Check sheet for the modelled part. Datum: model origin and axes. Units: mm. A direction names the side the tool comes from. Give positions to 0.01 mm unless a question says otherwise; leave off trailing zeros. Order: outer loops, then holes, each group sorted by start corner. A loop starts at its lowest first (then second) coordinate and runs counter-clockwise, first axis right, second up. Notation, with made-up numbers: (61, -35) - (76, -35) arc R10 ccw to (76, -26) - close; hole circle Ø4 at (28.5, 10.25). An arc over 180 degrees is marked (long way). Answer in a Markdown table with one row per item.
from build123d import *

# Parameters (mm, degrees)
SKETCH014_R     = 50
SKETCH014_R_2   = 31
SKETCH014_R_3   = 1.7
PAD014_DEPTH    = 8
SKETCH015_R     = 32.6
POCKET_DEPTH    = 7
SKETCH016_R     = 2.5
POCKET001_DEPTH = 7
SKETCH017_R     = 3
POCKET002_DEPTH = 4


with BuildPart() as part:
    # Sketch014 → Pad014 (new body)
    with BuildSketch(Plane.YZ):
        Circle(SKETCH014_R)
        Circle(SKETCH014_R_2, mode=Mode.SUBTRACT)
        with Locations((46, 0)):
            Circle(SKETCH014_R_3, mode=Mode.SUBTRACT)
        with Locations((-46, 0)):
            Circle(SKETCH014_R_3, mode=Mode.SUBTRACT)
        with Locations((0, -46)):
            Circle(SKETCH014_R_3, mode=Mode.SUBTRACT)
        with Locations((0, 46)):
            Circle(SKETCH014_R_3, mode=Mode.SUBTRACT)
        with Locations((-39.837169, 23)):
            Circle(SKETCH014_R_3, mode=Mode.SUBTRACT)
        with Locations((-23, 39.837169)):
            Circle(SKETCH014_R_3, mode=Mode.SUBTRACT)
        with Locations((39.837169, 23)):
            Circle(SKETCH014_R_3, mode=Mode.SUBTRACT)
        with Locations((39.837169, -23)):
            Circle(SKETCH014_R_3, mode=Mode.SUBTRACT)
        with Locations((23, -39.837169)):
            Circle(SKETCH014_R_3, mode=Mode.SUBTRACT)
        with Locations((23, 39.837169)):
            Circle(SKETCH014_R_3, mode=Mode.SUBTRACT)
        with Locations((-23, -39.837169)):
            Circle(SKETCH014_R_3, mode=Mode.SUBTRACT)
        with Locations((-39.837169, -23)):
            Circle(SKETCH014_R_3, mode=Mode.SUBTRACT)
    extrude(amount=PAD014_DEPTH)

    # Sketch015 (on DatumPlane) → Pocket (cut)
    with BuildSketch(Plane(origin=(0, 0, 0), x_dir=(0, 1, 0), z_dir=(-1, 0, 0))):
        Circle(SKETCH015_R)
    extrude(amount=-POCKET_DEPTH, mode=Mode.SUBTRACT)

    # Sketch016 (on DatumPlane) → Pocket001 (cut)
    with BuildSketch(Plane(origin=(0, 0, 0), x_dir=(0, 1, 0), z_dir=(-1, 0, 0))):
        with Locations((0, 35)):
            Circle(SKETCH016_R)
        with Locations((-35, 0)):
            Circle(SKETCH016_R)
        with Locations((0, -35)):
            Circle(SKETCH016_R)
        with Locations((35, 0)):
            Circle(SKETCH016_R)
        with Locations((24.748737, -24.748737)):
            Circle(SKETCH016_R)
        with Locations((-24.748737, -24.748737)):
            Circle(SKETCH016_R)
        with Locations((-24.748737, 24.748737)):
            Circle(SKETCH016_R)
        with Locations((24.748737, 24.748737)):
            Circle(SKETCH016_R)
    extrude(amount=-POCKET001_DEPTH, mode=Mode.SUBTRACT)

    # Sketch017 (on DatumPlane) → Pocket002 (cut)
    with BuildSketch(Plane.YZ.offset(8)):
        with Locations((-46, 0)):
            Circle(SKETCH017_R)
        with Locations((46, 0)):
            Circle(SKETCH017_R)
        with Locations((0, -46)):
            Circle(SKETCH017_R)
        with Locations((0, 46)):
            Circle(SKETCH017_R)
        with Locations((-39.837169, -23)):
            Circle(SKETCH017_R)
        with Locations((-23, -39.837169)):
            Circle(SKETCH017_R)
        with Locations((23, -39.837169)):
            Circle(SKETCH017_R)
        with Locations((39.837169, -23)):
            Circle(SKETCH017_R)
        with Locations((39.837169, 23)):
            Circle(SKETCH017_R)
        with Locations((23, 39.837169)):
            Circle(SKETCH017_R)
        with Locations((-23, 39.837169)):
            Circle(SKETCH017_R)
        with Locations((-39.837169, 23)):
            Circle(SKETCH017_R)
    extrude(amount=-POCKET002_DEPTH, mode=Mode.SUBTRACT)


solid = part.part
(1) Gauge pin test, flat ends, axial feed: P1, Ø3, axis at y = 24.75, z = -24.75, coming from the -X side; P2, Ø3, axis at x = 1, z = -28.5, coming from the +Y side; P3, Ø3, axis at y = -23, z = -39.5, coming from the +X side. Record the tip position at first contact, or that the pin passes through.
Geometry says:
| item | result |
|---|---|
| P1 | x = 7 |
| P2 | y = 42.08 |
| P3 | x = 4 |
(2) Thickness scan on L1, parallel to Y at x = 1.25, z = 39; L2, parallel to Z at x = 5.5, y = -38; L3, parallel to Y at x = 2, z = 25. Record the ranges inside material, lowest first.
Geometry says:
| item | result |
|---|---|
| L1 | -31.29 to -24.48, -21.52 to 21.52, 24.48 to 31.29 |
| L2 | -32.5 to -25.37, -20.63 to 20.63, 25.37 to 32.5 |
| L3 | -43.3 to -27.24, -22.26 to -20.92, 20.92 to 22.26, 27.24 to 43.3 |
(3) Mould release check, pull along Z, two halves, no side actions. Record for faces 4 (the flat face through (0, 10, -33)), 5 (the cylindrical face through (6, 0, 49)): pulls with the +Z half, pulls with the -Z half, needs draft (parallel to the pull), parting line crosses it, or undercut.
Geometry says:
| item | result |
|---|---|
| face 4 | needs draft |
| face 5 | undercut |
(4) Access from +Z, -Z, +X, -X, +Y, -Y to the whole of each face (thin tool, end or side, straight path). Record for faces 1 (the cylindrical face through (3.5, -0.1, 37.5)), 2 (the flat face through (4, 40, 21)), 3 (the cylindrical face through (1.97, 38.14, 23.07)).
Geometry says:
| item | result |
|---|---|
| face 1 | -X |
| face 2 | +X |
| face 3 | +X, -X |
(5) Cross-section at C-C, the plane x = 5.5. Give the number of separate pieces and of enclosed holes in the cut face, then the cut area to 3 significant figures.
Geometry says:
| item | result |
|---|---|
| separate pieces | 1 |
| enclosed holes | 13 |
| area | 4,020 mm² |
(6) Cross-section at A-A, the plane y = 46. Record the cut outline in (x, z), then the cut area to 3 significant figures.
Geometry says:
| item | result |
|---|---|
| outline | (0, -19.6) - (8, -19.6) - (8, -3) - (4, -3) - (4, -1.7) - (0, -1.7) - close; (0, 1.7) - (4, 1.7) - (4, 3) - (8, 3) - (8, 19.6) - (0, 19.6) - close |
| area | 276 mm² |
(7) Cross-section at D-D, the plane z = -35. Record the cut outline in (x, y).
Geometry says:
| item | result |
|---|---|
| outline | (0, -35.71) - (8, -35.71) - (8, 35.71) - (0, 35.71) - (0, 2.5) - (7, 2.5) - (7, -2.5) - (0, -2.5) - close |
(8) Cross-section at B-B, the plane z = 28.5. Record the cut outline in (x, y), then the cut area to 3 significant figures.
Geometry says:
| item | result |
|---|---|
| outline | (0, -41.08) - (8, -41.08) - (8, -12.2) - (7, -12.2) - (7, -15.83) - (0, -15.83) - close; (0, 15.83) - (7, 15.83) - (7, 12.2) - (8, 12.2) - (8, 41.08) - (0, 41.08) - close |
| area | 411 mm² |
